For this review, take the finished solid that the model builds, in its own axes (mm). A direction names the side the tool comes from. Round coordinates to 2 decimals unless told otherwise and drop trailing zeros. Order: outer loops, then holes, each group sorted by start corner. A loop starts at its lowest first (then second) coordinate and runs counter-clockwise, first axis right, second up. Notation, with made-up numbers: (-14.5, -39) - (32.5, -39) arc R18 cw to (32.5, -33) - close; hole circle Ø1 at (22, 31). An arc over 180 degrees is marked (long way). One line per question, with ' | ' between items.
```python
from build123d import *

# Parameters (mm, degrees)
F0_R     = 12.25
F1_DEPTH = 8.3
F2_R     = 6
F3_DEPTH = 8.301
F5_DEPTH = 4.3


with BuildPart() as f1:
    # F0 (on Right) → F1 (new body)
    with BuildSketch(Plane.YZ):
        Circle(F0_R)
    extrude(amount=F1_DEPTH)

    # F2 (on face) → F3 (cut, through all)
    with BuildSketch(Plane.YZ.offset(8.3)):
        Circle(F2_R)
    extrude(amount=-F3_DEPTH, mode=Mode.SUBTRACT)

    # F4 (on face) → F5 (cut)
    with BuildSketch(Plane(origin=(0, 0, 0), x_dir=(0, -1, 0), z_dir=(-1, 0, 0))):
        Polygon((4.907477, 8.5), (-4.907477, 8.5), (-9.814955, 0), (-4.907477, -8.5), (4.907477, -8.5), (9.814955, 0), align=None)
    extrude(amount=-F5_DEPTH, mode=Mode.SUBTRACT)


solid = f1.part
```
(1) We need section D-D on x = 6.25. State the section outline as (y, z) points.
Output values:
outline: circle Ø24.5 at (0, 0); hole circle Ø12 at (0, 0)
(2) We need section B-B on z = 1. State the section outline as (x, y) points.
Output values:
outline: (0, -12.21) - (8.3, -12.21) - (8.3, -5.92) - (4.3, -5.92) - (4.3, -9.24) - (0, -9.24) - close; (0, 9.24) - (4.3, 9.24) - (4.3, 5.92) - (8.3, 5.92) - (8.3, 12.21) - (0, 12.21) - close
(3) We need section A-A on y = 0. State the section outline as (x, z) points.
Output values:
outline: (0, -12.25) - (8.3, -12.25) - (8.3, -6) - (4.3, -6) - (4.3, -8.5) - (0, -8.5) - close; (0, 8.5) - (4.3, 8.5) - (4.3, 6) - (8.3, 6) - (8.3, 12.25) - (0, 12.25) - close
(4) For probe 1 along Z at (x, y) = (5.35, 0); probe 2 along Z at (x, y) = (3.75, -0.25); probe 3 along Y at (x, z) = (0.5, -8.25), list the stretches that pass through material, from the lowest coordinate up. Write a range as [from, to].
Output values:
probe 1: [-12.25, -6], [6, 12.25] | probe 2: [-12.25, -8.5], [8.5, 12.25] | probe 3: [-9.06, -5.05], [5.05, 9.06]
(5) For faces 1 (the flat face through (2.12, -7.396, 4.19)), 2 (the flat face through (8.3, 3, 6)), list the 3-axis set-ups (+Z, -Z, +X, -X, +Y, -Y) from which the entire face can be reached by the end or side of a thin tool; tool diameter is ignored.
Output values:
face 1: -X | face 2: +Z, -Z, +X, +Y, -Y
(6) Insertion check: pin 1 (1.3 mm diameter, centred on x = 2.5, y = -2, fed in from -Z); pin 2 (1.5 mm diameter, centred on x = 4, y = 2.5, fed in from +Z); pin 3 (12 mm diameter, centred on y = -6, z = 5, fed in from -X); pin 4 (2 mm diameter, centred on x = 1.5, y = 7, fed in from +Z). Each pin has a flat end and moves straight along its axis. Give the tip position at first contact, or say it passes through.
Output values:
pin 1: z = -12.18 | pin 2: z = 12.12 | pin 3: x = 0 | pin 4: z = 10.68
(7) Mouldability with a two-part tool opening along Y and no side actions: class faces 3 (the cylindrical face through (4.092, 6.586, 10.329)), 4 (the cylindrical face through (6, -6, 0)), 5 (the flat face through (0, 0, -9)) as released by +Y, released by -Y, zero draft, split by the parting line, or undercut.
Output values:
face 3: split by the parting line | face 4: undercut | face 5: zero draft
(8) We need section C-C on z = 8. State the section outline as (x, y) points.
Output values:
outline: (0, -9.28) - (8.3, -9.28) - (8.3, 9.28) - (0, 9.28) - (0, 5.2) - (4.3, 5.2) - (4.3, -5.2) - (0, -5.2) - close
